Geometry check sheet. Reference: the model listing, model coordinates, mm. A direction names the side the tool comes from. Coordinates: 2 decimals unless noted, no trailing zeros. Loops run counter-clockwise (first coordinate to the right, second up) from the corner with the lowest first, then second, coordinate; pieces in that order, holes last. Notation, with made-up numbers: (75, 69.25) - (88, 69.25) arc R31 cw to (88, 105.25) - close; hole circle Ø10 at (15, 86). An arc over 180 degrees is marked (long way). Write item = value, one per line. Start each with the question number.
from build123d import *

# Parameters (mm, degrees)
SKETCH1_W           = 51
SKETCH1_H           = 98
BOSS_EXTRUDE2_DEPTH = 3
BOSS_EXTRUDE3_DEPTH = 10
BOSS_EXTRUDE4_DEPTH = 10
SKETCH5_W           = 51
SKETCH5_H           = 1
BOSS_EXTRUDE5_DEPTH = 10
CUT_EXTRUDE1_DEPTH  = 10


with BuildPart() as part:
    # Sketch1 → Boss-Extrude2 (new body)
    with BuildSketch(Plane.XY):
        with Locations((25.5, 49)):
            Rectangle(SKETCH1_W, SKETCH1_H)
    extrude(amount=BOSS_EXTRUDE2_DEPTH)

    # Sketch3 → Boss-Extrude3 (add)
    with BuildSketch(Plane.XY.offset(3)):
        Polygon((0, 98), (7, 98), (7, 96), (2, 96), (2, 91), (0, 91), align=None)
        Polygon((51, 98), (44, 98), (44, 96), (49, 96), (49, 91), (51, 91), align=None)
        Polygon((51, 0), (44, 0), (44, 2), (49, 2), (49, 7), (51, 7), align=None)
    extrude(amount=BOSS_EXTRUDE3_DEPTH)

    # Sketch4 → Boss-Extrude4 (add)
    with BuildSketch(Plane.XY.offset(3)):
        Polygon((4, 0), (4, 7), (6, 7), (6, 2), (11.869482621, 2), (11.869482621, 0), align=None)
    extrude(amount=BOSS_EXTRUDE4_DEPTH)

    # Sketch5 → Boss-Extrude5 (add)
    with BuildSketch(Plane.XY.offset(3)):
        with Locations((25.5, 60.5)):
            Rectangle(SKETCH5_W, SKETCH5_H)
    extrude(amount=BOSS_EXTRUDE5_DEPTH)

    # Sketch6 → Cut-Extrude1 (cut)
    with BuildSketch(Plane.XY.offset(3)):
        Polygon((39.8, 93.770532131), (9.8, 93.770532131), (9.8, 68.770532131), (41.2, 68.770532131), (41.2, 93.770532131), align=None)
        Polygon((39.8, 50.5), (9.8, 50.5), (9.8, 10.5), (41.2, 10.5), (41.2, 50.5), align=None)
    extrude(amount=-CUT_EXTRUDE1_DEPTH, mode=Mode.SUBTRACT)


solid = part.part
(1) Depth check by flat-ended pin: pin 1 (5 mm diameter, centred on x = 38, z = 11, fed in from +Y); pin 2 (5.5 mm diameter, centred on y = 4.5, z = 6.5, fed in from -X). Enter the tip coordinate at first touch or a pass-through.
(2) Tool access check on faces 3 (the face through (44, 97, 8)), 4 (the face through (44, 1, 8)), 5 (the face through (7, 1, 13)), 6 (the face through (25, 10.5, 2)), 7 (the face through (49, 94, 8)). Record the directions out of +Z, -Z, +X, -X, +Y, -Y that give a thin tool (end or side, any length) a straight path to the whole face; none if there is none.
(3) Draft check along X on faces 1 (the face through (26, 50.5, 2)), 2 (the face through (50, 7, 8)). Enter one of: pulls with the +X half, pulls with the -X half, needs draft (parallel to the pull), parting line crosses it, or undercut.
(4) Sectioned sample at C-C on x = 22. Enter the section's corners in (y, z).
(5) Scan lines: line 1 (Y direction, x = 48.5, z = 5.5); line 2 (X direction, y = 21, z = 1); line 3 (X direction, y = 4.5, z = 8.5). Record each from-to range of solid material in increasing order.
(6) Sectioned sample at D-D on z = 1.75. Enter the section's corners in (x, y), plus the area to 3 significant figures.
(7) Sectioned sample at B-B on y = 25.5. Enter the section's corners in (x, z), plus the area to 3 significant figures.
(8) Sectioned sample at A-A on z = 6.75. Enter the section's corners in (x, y), plus the area to 3 significant figures.
Working result:
q1.pin_1 = 61
q1.pin_2 = 4
q2.face_3 = +Z, +Y
q2.face_4 = +Z, -Y
q2.face_5 = +Z, +X, -X, +Y, -Y
q2.face_6 = +Z, -Z
q2.face_7 = +Z
q3.face_1 = undercut
q3.face_2 = needs draft
q4.outline = (0, 0) - (10.5, 0) - (10.5, 3) - (0, 3) - close; (50.5, 0) - (68.77, 0) - (68.77, 3) - (61, 3) - (61, 13) - (60, 13) - (60, 3) - (50.5, 3) - close; (93.77, 0) - (98, 0) - (98, 3) - (93.77, 3) - close
q5.line_1 = 0 to 2, 60 to 61, 96 to 98
q5.line_2 = 0 to 9.8, 41.2 to 51
q5.line_3 = 4 to 6, 49 to 51
q6.outline = (0, 0) - (51, 0) - (51, 98) - (0, 98) - close; hole (9.8, 10.5) - (41.2, 10.5) - (41.2, 50.5) - (9.8, 50.5) - close; hole (9.8, 68.77) - (41.2, 68.77) - (41.2, 93.77) - (9.8, 93.77) - close
q6.area = 2,960 mm2
q7.outline = (0, 0) - (9.8, 0) - (9.8, 3) - (0, 3) - close; (41.2, 0) - (51, 0) - (51, 3) - (41.2, 3) - close
q7.area = 58.8 mm2
q8.outline = (0, 60) - (51, 60) - (51, 61) - (0, 61) - close; (0, 91) - (2, 91) - (2, 96) - (7, 96) - (7, 98) - (0, 98) - close; (4, 0) - (11.87, 0) - (11.87, 2) - (6, 2) - (6, 7) - (4, 7) - close; (44, 0) - (51, 0) - (51, 7) - (49, 7) - (49, 2) - (44, 2) - close; (44, 96) - (49, 96) - (49, 91) - (51, 91) - (51, 98) - (44, 98) - close
q8.area = 149 mm2
